Model file for the job. Use its own axes, mm. Round coordinates to 2 decimals unless told otherwise and drop trailing zeros. Order: outer loops, then holes, each group sorted by start corner. A loop starts at its lowest first (then second) coordinate and runs counter-clockwise, first axis right, second up. Notation, with made-up numbers: (47.5, 77.25) -> (97.5, 77.25) arc R21 cw to (97.5, 82.25) -> close; hole circle Ø1 at (65.25, -3.5). An arc over 180 degrees is marked (long way). Put each result on its own line as item: value. Start each with the question number.
Q1. Flat gauge pins, fed straight in: P1, Ø10, axis at y = -26.5, z = 54.5, coming from the -X side; P2, Ø1, axis at x = -22, z = 21.5, coming from the +Y side; P3, Ø10, axis at y = -31, z = -65, coming from the -X side. Where does each tip first touch, or does it go through?
Q2. Cut at C-C, the plane z = -28.5. List the corners of the cut face in (x, y), and give its area (3 significant figures).
Q3. Pull direction X, two halves, no side cores. Call faces 1 (the face through (-28.933, 26.531, 2.845)), 2 (the face through (-32, 21, -203.2)), 3 (the face through (-30.235, -23.183, -2.845)): released by +X, released by -X, zero draft, split by the parting line, or undercut.
Q4. Probe L1, parallel to Y at x = 0, z = -24; L2, parallel to Y at x = 7.5, z = -150.5. List the from-to ranges inside material, lowest first.
Q5. Cut at B-B, the plane y = -33. List the corners of the cut face in (x, z), and give its area (3 significant figures).
Q6. Cut at A-A, the plane x = -8.5. List the corners of the cut face in (y, z), and give its area (3 significant figures).
from build123d import *

# Parameters (mm, degrees)
SKETCH1_R           = 39.2557
SKETCH1_R_2         = 38.1
BOSS_EXTRUDE1_DEPTH = 203.2
SKETCH3_W           = 3.175
SKETCH3_H           = 127
CUT_EXTRUDE1_DEPTH  = 40.2557
CIRPATTERN1_COUNT   = 4


with BuildPart() as part:
    # Sketch1 → Boss-Extrude1 (new body, symmetric)
    with BuildSketch(Plane.XY):
        Circle(SKETCH1_R)
        Circle(SKETCH1_R_2, mode=Mode.SUBTRACT)
    extrude(amount=BOSS_EXTRUDE1_DEPTH, both=True)

    # Sketch3 → Cut-Extrude1 (cut, through all)
    with BuildSketch(Plane(origin=(0, 0, 0), x_dir=(1, 0, 0), z_dir=(0, 1, 0))):
        with Locations((0, 120.65)):
            Rectangle(SKETCH3_W, SKETCH3_H)
    cut_extrude1 = extrude(amount=CUT_EXTRUDE1_DEPTH, mode=Mode.SUBTRACT)

    # CirPattern1: Cut-Extrude1 ×4 about axis
    cirpattern1_axis = Axis((0, 0, 0), (0, 0, 1))
    for i in range(1, CIRPATTERN1_COUNT):
        add(cut_extrude1.rotate(cirpattern1_axis, i * 360 / CIRPATTERN1_COUNT), mode=Mode.SUBTRACT)


solid = part.part
Ans:
1. P1: stops at x = -32.84
1. P2: stops at y = 32.84
1. P3: stops at x = -29.41
2. outline: circle Ø78.51 at (0, 0); hole circle Ø76.2 at (0, 0)
2. area: 281 mm^2
3. face 1: split by the parting line
3. face 2: zero draft
3. face 3: undercut
4. L1: y = -39.26 to -38.1, 38.1 to 39.26
4. L2: y = -38.53 to -37.35, 37.35 to 38.53
5. outline: (-21.26, -203.2) -> (-19.04, -203.2) -> (-19.04, 203.2) -> (-21.26, 203.2) -> close; (19.04, -203.2) -> (21.26, -203.2) -> (21.26, 203.2) -> (19.04, 203.2) -> close
5. area: 1,800 mm^2
6. outline: (-38.32, -203.2) -> (-37.14, -203.2) -> (-37.14, 203.2) -> (-38.32, 203.2) -> close; (37.14, -203.2) -> (38.32, -203.2) -> (38.32, 203.2) -> (37.14, 203.2) -> close
6. area: 963 mm^2
